Autodesk Inventor part; units mm, degrees
ref_plane "YZ Plane" through (0, 0, 0) normal (1, 0, 0) x (0, 1, 0)
ref_plane "XZ Plane" through (0, 0, 0) normal (0, 1, 0) x (-1, 0, 0)
ref_plane "XY Plane" through (0, 0, 0) normal (0, 0, 1) x (1, 0, 0)
sketch "スケッチ1" plane through (0, 0, 0) normal (1, 0, 0) x (0, 1, 0)
  line L0 (0, 0) -> (1, 0) construction
  line L1 (1.9, 0) -> (1.9, 1.75)
  line L2 (1.65, 2) -> (0.866, 2)
  line L3 (0, 2) -> (0, 1.5) construction
  line L4 (1, 0) -> (1, -4)
  line L5 (1, -4) -> (0, -4)
  line L6 (0, -4) -> (0, 0)
  line L7 (1, 0) -> (1.9, 0)
  line L8 (0.866, 2) -> (0.433, 1.25) construction
  line L9 (0.433, 1.25) -> (-0.433, 1.25) construction
  line L10 (-0.433, 1.25) -> (-0.866, 2) construction
  line L11 (-0.866, 2) -> (-0.433, 2.75) construction
  line L12 (-0.433, 2.75) -> (0.433, 2.75) construction
  line L13 (0.433, 2.75) -> (0.866, 2) construction
  line L14 (0.866, 2) -> (0, 1.5)
  line L15 (0.866, 2) -> (0, 2) construction
  line L16 (0, 1.5) -> (0, 0)
  arc A0 (1.9, 1.75) -> (1.65, 2) centre (1.65, 1.75) ccw
  dimension "d0" = 1.5
  dimension "d1" = 3.8
  dimension "d2" = 2
  dimension "d3" = 4
  dimension "d4" = 2
  dimension "d6" = 0.25
  dimension "d11" = 30
revolve "回転1" add sketch "スケッチ1" angle 360 about axis through (0, 0, 1.5) along (0, 0, -1)
sketch "スケッチ2" plane through (0, 0, 2) normal (0, 0, 1) x (1, 0, 0)
  line L0 (0.866, 0) -> (0.433, -0.75)
  line L1 (0.433, -0.75) -> (-0.433, -0.75)
  line L2 (-0.433, -0.75) -> (-0.866, 0)
  line L3 (-0.866, 0) -> (-0.433, 0.75)
  line L4 (-0.433, 0.75) -> (0.433, 0.75)
  line L5 (0.433, 0.75) -> (0.866, 0)
  point P0 (0, 0)
  point P1 (0, 0)
  dimension "d8" = 1.5
extrude "押し出し1" cut sketch "スケッチ2" against normal blind 1
chamfer "面取り1" distance 0.25 angle 45 1 edges at (0, -1, -4)
properties part number "10_048_CAP_SCREW_M2X4_R1" material "鋼、炭素鋼"
Can you work these out from the model? Positions are in its coordinate system, mm. A direction names the side the tool comes from. Coordinates: 2 decimals unless noted, no trailing zeros. Write each loop counter-clockwise with the first axis right and the second up, starting at its lowest first coordinate (ties: lowest second). Pieces come first, ordered by that corner, then holes.
Q1. Imagine slicing it at C-C, the plane z = -2.5. List the corners of the cut face in (x, y) for me, plus the area to 3 significant figures.
Results found:
outline: circle Ø2 at (0, 0)
area: 3.14 mm2
Q2. If we mould it in two halves opening along Y, with no side actions, what happens to faces 4 (the face through (0, -0.75, 1.5)), 5 (the face through (0, 0, -4)), 6 (the face through (-1, 0, -2))? For each: +Y half, -Y half, draft (parallel to the pull), parting line (faces both ways), or undercut.
Results found:
face 4: undercut
face 5: draft
face 6: parting line
Q3. Please list where these lines run through material, in increasing order: L1, parallel to Z at x = 0.3, y = 1.55; L2, parallel to Z at x = 0.45, y = 0.45; L3, parallel to X at y = 0, z = -3.5.
Results found:
L1: z = 0 to 2
L2: z = -4 to 1
L3: x = -1 to 1
Q4. Imagine slicing it at D-D, the plane z = 0.5. List the corners of the cut face in (x, y) for me, plus the area to 3 significant figures.
Results found:
outline: circle Ø3.8 at (0, 0)
area: 11.3 mm2
Q5. Imagine slicing it at A-A, the plane z = 1.25. List the corners of the cut face in (x, y) for me.
Results found:
outline: circle Ø3.8 at (0, 0); hole (-0.87, 0) - (-0.43, -0.75) - (0.43, -0.75) - (0.87, 0) - (0.43, 0.75) - (-0.43, 0.75) - close
Q6. Imagine slicing it at B-B, the plane x = 0. List the corners of the cut face in (y, z) for me.
Results found:
outline: (-1.9, 0) - (-1, 0) - (-1, -3.75) - (-0.75, -4) - (0.75, -4) - (1, -3.75) - (1, 0) - (1.9, 0) - (1.9, 1.75) arc R0.25 ccw to (1.65, 2) - (0.87, 2) - (0.75, 1.93) - (0.75, 1) - (-0.75, 1) - (-0.75, 1.93) - (-0.87, 2) - (-1.65, 2) arc R0.25 ccw to (-1.9, 1.75) - close
Q7. Which directions (+Z, -Z, +X, -X, +Y, -Y) give clear straight access to the entire face, cutting with the end or side of a thin tool? Please do faces 1 (the face through (-1, 1, 0)), 2 (the face through (-0.08, -1.9, 0.89)), 3 (the face through (0, 0, 1)).
Results found:
face 1: -Z
face 2: +Z, -Z
face 3: +Z
Q8. For P1, Ø1.5, axis at x = -0.5, z = -1.5, coming from the +Y side, with a flat end and sliding along its axis, tell me the tip position at first contact or that it passes through.
Results found:
P1: stops at y = 1
